```python
from build123d import *

# Parameters (mm, degrees)
F0_R     = 19.05
F0_R_2   = 15.875
F1_DEPTH = 254
F2_R     = 25.4
F2_R_2   = 6.35
F3_DEPTH = 25.4
F4_R     = 25.4
F4_R_2   = 12.7
F5_DEPTH = 25.4
F7_D     = 12.7
F7_DEPTH = 25.401


with BuildPart() as f1:
    # F0 (on Front) → F1 (new body)
    with BuildSketch(Plane.XZ):
        Circle(F0_R)
        Circle(F0_R_2, mode=Mode.SUBTRACT)
    extrude(amount=F1_DEPTH)

    # F2 (on face) → F3 (join)
    with BuildSketch(Plane(origin=(0, 0, 0), x_dir=(-1, 0, 0), z_dir=(0, 1, 0))):
        Circle(F2_R)
        Circle(F2_R_2, mode=Mode.SUBTRACT)
    extrude(amount=F3_DEPTH)

    # F4 (on face) → F5 (join)
    with BuildSketch(Plane.XZ.offset(254)):
        Circle(F4_R)
        Circle(F4_R_2, mode=Mode.SUBTRACT)
    extrude(amount=F5_DEPTH)

    # F7 (through all, one way)
    with BuildSketch(Plane.YZ):
        with Locations((-228.6, 0)):
            Circle(F7_D / 2)
    extrude(amount=-F7_DEPTH, mode=Mode.SUBTRACT)


solid = f1.part
```
The model under review builds one solid part; all positions refer to its coordinate system, in mm. A direction names the side the tool comes from. Round coordinates to 2 decimals unless told otherwise and drop trailing zeros. Loops run counter-clockwise (first coordinate to the right, second up) from the corner with the lowest first, then second, coordinate; pieces in that order, holes last. Notation, with made-up numbers: (39.25, -33) -> (52.25, -33) arc R27 cw to (52.25, 4) -> close; hole circle Ø1 at (-8.5, -17.5). An arc over 180 degrees is marked (long way). Answer in a Markdown table with one row per item.
1) Consider section C-C, the plane y = -205.5. Write out the cut boundary in (x, z) (3 decimals), plus the area to 3 significant figures.
Taken from the geometry:
| item | result |
|---|---|
| outline | circle Ø38.1 at (0, 0); hole circle Ø31.75 at (0, 0) |
| area | 348 mm² |
2) Consider section B-B, the plane z = 0. Write out the cut boundary in (x, y) (3 decimals).
Taken from the geometry:
| item | result |
|---|---|
| outline | (-25.4, -279.4) -> (-12.7, -279.4) -> (-12.7, -254) -> (-15.875, -254) -> (-15.875, -234.95) -> (-19.05, -234.95) -> (-19.05, -254) -> (-25.4, -254) -> close; (-25.4, 0) -> (-19.05, 0) -> (-19.05, -222.25) -> (-15.875, -222.25) -> (-15.875, 0) -> (-6.35, 0) -> (-6.35, 25.4) -> (-25.4, 25.4) -> close; (6.35, 0) -> (15.875, 0) -> (15.875, -254) -> (12.7, -254) -> (12.7, -279.4) -> (25.4, -279.4) -> (25.4, -254) -> (19.05, -254) -> (19.05, 0) -> (25.4, 0) -> (25.4, 25.4) -> (6.35, 25.4) -> close |
3) Tool access review of faces 1 (the cylindrical face through (-3.441, -125.222, -15.497)), 2 (the cylindrical face through (5.506, 12.522, -24.796)), 3 (the cylindrical face through (-2.75, -266.52, -12.4)), 4 (the cylindrical face through (-16.768, -222.543, 1.907)), 5 (the flat face through (-5, 25.4, -5)): name each direction out of +Z, -Z, +X, -X, +Y, -Y from which nothing blocks a thin tool from reaching the whole face with its end or side.
Taken from the geometry:
| item | result |
|---|---|
| face 1 | none |
| face 2 | +Y, -Y |
| face 3 | -Y |
| face 4 | -X |
| face 5 | +Z, -Z, +X, -X, +Y |
4) Consider section A-A, the plane x = 0. Write out the cut boundary in (y, z) (3 decimals), plus the area to 3 significant figures.
Taken from the geometry:
| item | result |
|---|---|
| outline | (-279.4, -25.4) -> (-254, -25.4) -> (-254, -19.05) -> (0, -19.05) -> (0, -25.4) -> (25.4, -25.4) -> (25.4, -6.35) -> (0, -6.35) -> (0, -15.875) -> (-254, -15.875) -> (-254, -12.7) -> (-279.4, -12.7) -> close; (-279.4, 12.7) -> (-254, 12.7) -> (-254, 15.875) -> (0, 15.875) -> (0, 6.35) -> (25.4, 6.35) -> (25.4, 25.4) -> (0, 25.4) -> (0, 19.05) -> (-254, 19.05) -> (-254, 25.4) -> (-279.4, 25.4) -> close |
| area | 3,230 mm² |
5) Wall thickness on line 1 along Z through (x, y) = (0, -274.5); line 2 along X through (y, z) = (-147, 0) (3 decimals); line 3 along Y through (x, z) = (12.5, 8): over which ranges is each line inside the solid? List them lowest first.
Taken from the geometry:
| item | result |
|---|---|
| line 1 | z = -25.4 to -12.7, 12.7 to 25.4 |
| line 2 | x = -19.05 to -15.875, 15.875 to 19.05 |
| line 3 | y = -279.4 to -254, 0 to 25.4 |
6) For pin 1 Ø4 at (x, z) = (-6, -0.5) entering from -Y; pin 2 Ø10 at (x, y) = (13.5, -234) entering from +Z; pin 3 Ø3 at (x, y) = (-3.5, -77) entering from -Z; pin 4 Ø7.5 at (x, z) = (0, 0) entering from +Y, all flat-tipped, find the tip position at first contact; note any pin that passes through.
Taken from the geometry:
| item | result |
|---|---|
| pin 1 | stops at y = 0 |
| pin 2 | stops at z = 17.05 |
| pin 3 | stops at z = -18.94 |
| pin 4 | passes through |
7) Draft analysis for pull direction Y (two halves, no side actions). For faces 6 (the flat face through (-4, 0, 19)), 7 (the flat face through (-7, 0, 0)), 8 (the cylindrical face through (1.38, 12.52, -6.2)), 9 (the flat face through (5, -279.4, 12)), state which applies: pulls with the +Y half, pulls with the -Y half, needs draft (parallel to the pull), parting line crosses it, or undercut.
Taken from the geometry:
| item | result |
|---|---|
| face 6 | undercut |
| face 7 | undercut |
| face 8 | needs draft |
| face 9 | pulls with the -Y half |
